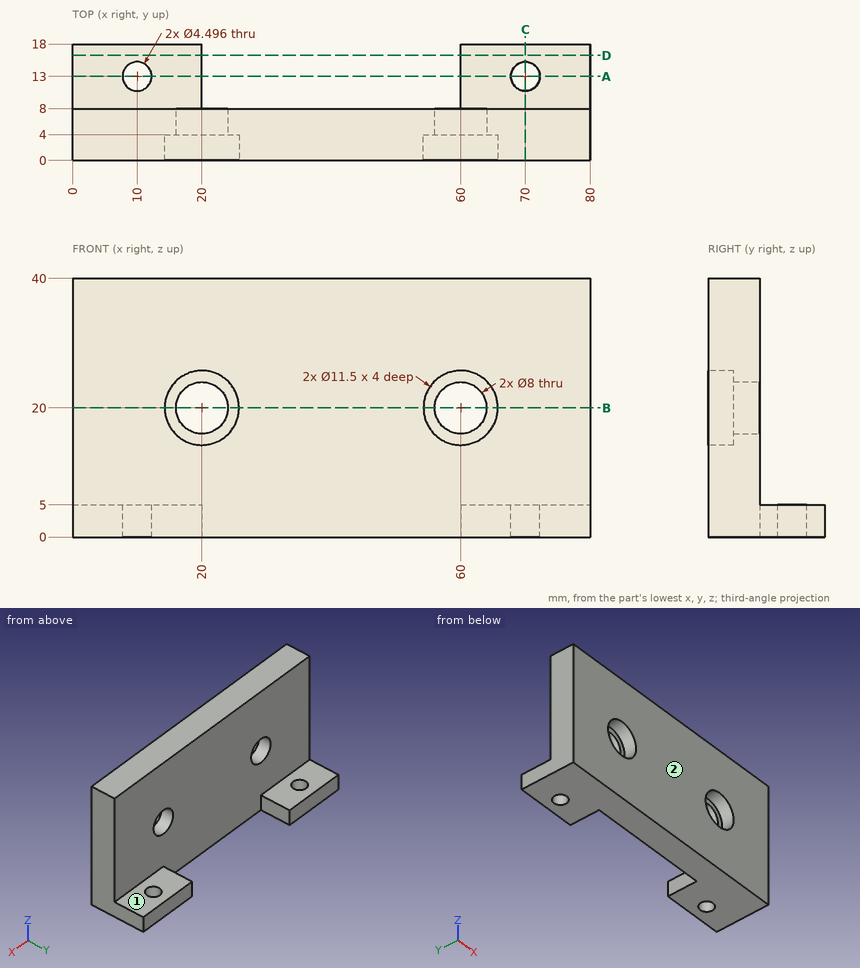
Study the drawing (mm; zero at the part's minimum x, y, z) and answer. A direction names the side the tool comes from. Give positions to 0.01 mm unless a question says otherwise; leave off trailing zeros. Order: outer loops, then holes, each group sorted by start corner. A loop starts at its lowest first (then second) coordinate and runs counter-clockwise, first axis right, second up.
1) Find section D-D on y = 16.25. Write down the section's boundary in (x, z), then the cut area to 3 significant figures.
Reported:
outline: (0, 0) - (20, 0) - (20, 5) - (0, 5) - close; (60, 0) - (80, 0) - (80, 5) - (60, 5) - close
area: 200 mm2
2) Consider line 1 along X through (y, z) = (1.9, 20); line 2 along Z through (x, y) = (60, 3.25); line 3 along Y through (x, z) = (10, 2.3). Determine where each line is inside the solid, lowest interval first.
Reported:
line 1: x = 0 to 14.25, 25.75 to 54.25, 65.75 to 80
line 2: z = 0 to 14.25, 25.75 to 40
line 3: y = 0 to 10.75, 15.25 to 18
3) Find section C-C on x = 70. Write down the section's boundary in (y, z).
Reported:
outline: (0, 0) - (10.75, 0) - (10.75, 5) - (8, 5) - (8, 40) - (0, 40) - close; (15.25, 0) - (18, 0) - (18, 5) - (15.25, 5) - close
4) For the marked faces 1 and 2, determine the directions among +Z, -Z, +X, -X, +Y, -Y from which every point of the face is accessible in a straight line to the end or side of a thin tool.
Reported:
face 1: +Z, +X, -X, +Y
face 2: +Z, -Z, +X, -X, -Y
5) Find section B-B on z = 20. Write down the section's boundary in (x, y), then the cut area to 3 significant figures.
Reported:
outline: (0, 0) - (14.25, 0) - (14.25, 4) - (16, 4) - (16, 8) - (0, 8) - close; (24, 4) - (25.75, 4) - (25.75, 0) - (54.25, 0) - (54.25, 4) - (56, 4) - (56, 8) - (24, 8) - close; (64, 4) - (65.75, 4) - (65.75, 0) - (80, 0) - (80, 8) - (64, 8) - close
area: 484 mm2
6) Given P1, Ø12, axis at x = 20, z = 17, coming from the +Y side; P2, Ø6, axis at x = 59.5, z = 21.5, coming from the -Y side; P3, Ø5, axis at x = 73.5, y = 13, coming from the +Z side; P4, Ø5, axis at x = 20, z = 20, coming from the -Y side, each flat-ended and moving along its own axis, determine where each tip first touches the part or whether it passes through.
Reported:
P1: stops at y = 8
P2: stops at y = 4
P3: stops at z = 5
P4: passes through
7) Find section A-A on y = 13. Write down the section's boundary in (x, z), then the cut area to 3 significant figures.
Reported:
outline: (0, 0) - (7.75, 0) - (7.75, 5) - (0, 5) - close; (12.25, 0) - (20, 0) - (20, 5) - (12.25, 5) - close; (60, 0) - (67.75, 0) - (67.75, 5) - (60, 5) - close; (72.25, 0) - (80, 0) - (80, 5) - (72.25, 5) - close
area: 155 mm2
